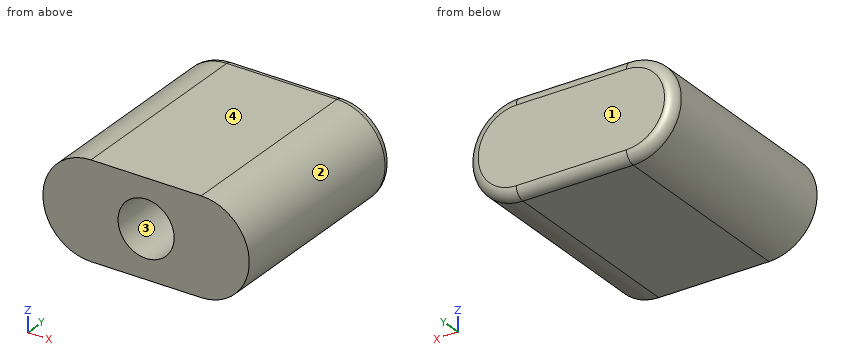
from build123d import *

# Parameters (mm, degrees)
BOSS_EXTRUDE1_DEPTH = 13.335
FILLET1_R           = 0.635
SKETCH2_R           = 1.778
CUT_EXTRUDE3_DEPTH  = 6.985


with BuildPart() as part:
    # Sketch1 → Boss-Extrude1 (new body)
    with BuildSketch(Plane(origin=(0, 0, 0), x_dir=(1, 0, 0), z_dir=(0, 1, 0))):
        with BuildLine():
            Line((-3.4925, 3.048), (3.4925, 3.048))
            ThreePointArc((3.4925, 3.048), (6.5405, 0), (3.4925, -3.048))
            Line((3.4925, -3.048), (-3.4925, -3.048))
            ThreePointArc((-3.4925, -3.048), (-6.5405, 0), (-3.4925, 3.048))
        make_face()
    extrude(amount=BOSS_EXTRUDE1_DEPTH)

    # Fillet1
    fillet1_edges = [part.edges().sort_by_distance(p)[0] for p in [
        (6.5405, 13.335, 0),
        (0, 13.335, -3.048),
        (-6.5405, 13.335, 0),
        (0, 13.335, 3.048),
    ]]
    fillet(fillet1_edges, radius=FILLET1_R)

    # Sketch2 → Cut-Extrude3 (cut)
    with BuildSketch(Plane.XZ):
        Circle(SKETCH2_R)
    extrude(amount=-CUT_EXTRUDE3_DEPTH, mode=Mode.SUBTRACT)


solid = part.part
Can you work these out from the model? Positions are in its coordinate system, mm. Face numbers are marked on the shaded views. Round coordinates to 2 decimals unless told otherwise and drop trailing zeros. Write each loop counter-clockwise with the first axis right and the second up, starting at its lowest first coordinate (ties: lowest second). Pieces come first, ordered by that corner, then holes. Notation, with made-up numbers: M 8,-8.75 L 49,-8.75 A19 cw 49,28.25 Z; hole C 36.5,34 d7. An arc over 180 degrees is marked long. Use a Markdown table: item, result.
Item 1: We'd pull the mould along Z, two halves only. Please class the marked faces 1, 2, 3 and 4: released by +Z, released by -Z, zero draft, split by the parting line, or undercut.
Found:
| item | result |
|---|---|
| face 1 | zero draft |
| face 2 | split by the parting line |
| face 3 | undercut |
| face 4 | released by +Z |
Item 2: I want a section at A-A (x = 0). List the corners of the cut face in (y, z) for me (3 decimals).
Found:
| item | result |
|---|---|
| outline | M 0,-3.048 L 12.7,-3.048 A0.635 ccw 13.335,-2.413 L 13.335,2.413 A0.635 ccw 12.7,3.048 L 0,3.048 L 0,1.778 L 6.985,1.778 L 6.985,-1.778 L 0,-1.778 Z |
Item 3: I want a section at D-D (y = 10.25). List the corners of the cut face in (x, z) for me.
Found:
| item | result |
|---|---|
| outline | M -3.49,-3.05 L 3.49,-3.05 A3.05 ccw 3.49,3.05 L -3.49,3.05 A3.05 ccw Z |
Item 4: I want a section at B-B (y = 5.25). List the corners of the cut face in (x, z) for me, and give its area (3 significant figures).
Found:
| item | result |
|---|---|
| outline | M -3.49,-3.05 L 3.49,-3.05 A3.05 ccw 3.49,3.05 L -3.49,3.05 A3.05 ccw Z; hole C 0,0 d3.56 |
| area | 61.8 mm2 |
Item 5: I want a section at C-C (z = 0). List the corners of the cut face in (x, y) for me (1 decimal), and give its area (3 significant figures).
Found:
| item | result |
|---|---|
| outline | M -6.5,0 L -1.8,0 L -1.8,7 L 1.8,7 L 1.8,0 L 6.5,0 L 6.5,12.7 A0.6 ccw 5.9,13.3 L -5.9,13.3 A0.6 ccw -6.5,12.7 Z |
| area | 149 mm2 |
Item 6: If I drill on line 1 along Z through (x, y) = (0, 2.25); line 2 along Y through (x, z) = (-1, -0.75) (3 decimals); line 3 along Z through (x, y) = (1.25, 5), over which ranges is the centre line in solid material (lowest first)? Write a range as [from, to].
Found:
| item | result |
|---|---|
| line 1 | z = [-3.05, -1.78], [1.78, 3.05] |
| line 2 | y = [6.985, 13.335] |
| line 3 | z = [-3.05, -1.26], [1.26, 3.05] |
